Autodesk Inventor part; units mm, degrees
ref_plane "YZ Plane" through (0, 0, 0) normal (1, 0, 0) x (0, 1, 0)
ref_plane "XZ Plane" through (0, 0, 0) normal (0, 1, 0) x (-1, 0, 0)
ref_plane "XY Plane" through (0, 0, 0) normal (0, 0, 1) x (1, 0, 0)
sketch "Block1" plane through (0, 0, 0) normal (0, 0, 1) x (1, 0, 0)
  circle A0 centre (74.029, 24.2723) radius 1
  line L0 (49.279, 30.4723) -> (71.779, 30.4723)
  line L1 (71.779, 30.4723) -> (71.779, 18.0723)
  line L2 (71.779, 18.0723) -> (49.279, 18.0723)
  line L3 (49.279, 18.0723) -> (49.279, 30.4723)
  line L4 (49.279, 30.4723) -> (44.779, 30.4723)
  line L5 (44.779, 30.4723) -> (44.779, 18.0723)
  line L6 (44.779, 18.0723) -> (49.279, 18.0723)
  line L7 (49.279, 18.0723) -> (49.279, 30.4723)
  line L8 (71.779, 30.4723) -> (76.279, 30.4723)
  line L9 (76.279, 30.4723) -> (76.279, 18.0723)
  line L10 (76.279, 18.0723) -> (71.779, 18.0723)
  line L11 (71.779, 18.0723) -> (71.779, 30.4723)
  line L12 (44.779, 24.2723) -> (76.279, 24.2723) construction
  line L13 (47.029, 30.4723) -> (47.029, 18.0723) construction
  circle A1 centre (47.029, 24.2723) radius 1
  line L14 (74.029, 30.4723) -> (74.029, 18.0723) construction
  point P0 (60.979, 24.0984)
  dimension "d7" = 22.5
  dimension "d8" = 12.4
  dimension "d9" = 4.5
  dimension "d10" = 4.5
  dimension "d11" = 2
  dimension "d12" = 2
sketch "Sketch1" plane through (0, 0, 0) normal (0, 0, 1) x (1, 0, 0)
  line L0 (-92.7646, -8.503) -> (-89.7646, -8.503)
  line L1 (-89.7646, -8.503) -> (-89.7646, -11.753)
  line L2 (-89.7646, -11.753) -> (-92.7646, -11.753)
  line L3 (-92.7646, -11.753) -> (-92.7646, -8.503)
  line L4 (-92.7646, -21.6527) -> (-89.7646, -21.6527)
  line L5 (-89.7646, -21.6527) -> (-89.7646, -21.7527)
  line L6 (-89.7646, -21.7527) -> (-92.7646, -21.7527)
  line L7 (-92.7646, -21.7527) -> (-92.7646, -21.6527)
  line L8 (-51.3097, 52.8088) -> (28.6903, 52.8088)
  line L9 (28.6903, 52.8088) -> (28.6903, 26.8088)
  line L10 (28.6903, 26.8088) -> (-51.3097, 26.8088)
  line L11 (-51.3097, 26.8088) -> (-51.3097, 52.8088)
  line L12 (-51.3097, 39.8088) -> (28.6903, 39.8088) construction
  line L13 (-21.3097, 46.8088) -> (-18.0597, 46.8088)
  line L14 (-18.0597, 46.8088) -> (-18.0597, 32.8088)
  line L15 (-18.0597, 32.8088) -> (-21.3097, 32.8088)
  line L16 (-21.3097, 32.8088) -> (-21.3097, 46.8088)
  line L17 (-21.3097, 39.8088) -> (-18.0597, 39.8088) construction
  line L18 (-38.3097, 52.8088) -> (-38.3097, 26.8088) construction
  arc A0 (-38.3097, 52.8088) -> (-38.3097, 26.8088) centre (-38.3097, 39.8088) ccw
  line L19 (-11.3097, 52.8088) -> (-11.3097, 26.8088) construction
  line L20 (15.6903, 52.8088) -> (15.6903, 26.8088) construction
  arc A1 (15.6903, 26.8088) -> (15.6903, 52.8088) centre (15.6903, 39.8088) ccw
  point P0 (0, 0)
  dimension "d0" = 3
  dimension "mat" = 3.25
  dimension "d2" = 3
  dimension "d3" = 0.1
  dimension "d23" = 80
  dimension "d24" = 26
  dimension "d29" = 3.25
  dimension "d30" = 14
  dimension "d31" = 30
  dimension "d38" = 13
  dimension "d39" = 13
extrude "Extrusion6" add sketch "Sketch1" along normal blind 3.25 contours L8 A1 L10 A0
equation "\"d29\" = mat"
equation "\"d42\" = mat"
properties part number "arm-servo"
CAD build for the part. Positions are in the model's coordinates, mm. A direction names the side the tool comes from. Give positions to 0.01 mm unless a question says otherwise; leave off trailing zeros. Order: outer loops, then holes, each group sorted by start corner. A loop starts at its lowest first (then second) coordinate and runs counter-clockwise, first axis right, second up.
(1) Saw through at C-C, the plane x = 22.5. Give the cut face in (y, z).
(2) Flat gauge pins, fed straight in: pin 1 (1 mm diameter, centred on y = 41.5, z = 3, fed in from +X); pin 2 (1.6 mm diameter, centred on y = 43, z = 1, fed in from +X); pin 3 (1 mm diameter, centred on y = 41.5, z = 1.5, fed in from -X) (3 decimals). Where does each tip first touch, or does it go through?
(3) Tool access for faces 4 (the flat face through (-12, 40, 0)), 5 (the flat face through (-21.31, 40, 2)): list every direction of +Z, -Z, +X, -X, +Y, -Y with a clear straight run to the whole face (end or side of a thin tool).
(4) Mould opens along Y. For faces 1 (the flat face through (-18.06, 40, 2)), 2 (the cylindrical face through (28.687, 40.095, 1.602)), 3 (the flat face through (-11, 26.809, 2)) say: released by +Y, released by -Y, zero draft, split by the parting line, or undercut.
(5) Drill centre lines: L1, parallel to X at y = 35.5, z = 2.15; L2, parallel to X at y = 45, z = 1.5; L3, parallel to X at y = 50.5, z = 1.15. Where is each one in solid material? Low to high.
(6) Saw through at A-A, the plane z = 2.4. Give the cut face in (x, y).
(7) Saw through at D-D, the plane y = 39.25. Give the cut face in (x, z), then the cut area to 3 significant figures.
(8) Saw through at B-B, the plane y = 43. Give the cut face in (x, z).
Results found:
1. outline: (28.74, 0) - (50.88, 0) - (50.88, 3.25) - (28.74, 3.25) - close
2. pin 1: stops at x = 28.64
2. pin 2: stops at x = 28.47
2. pin 3: stops at x = -51.255
3. face 4: -Z, +X, -X, +Y, -Y
3. face 5: +Z, -Z
4. face 1: undercut
4. face 2: split by the parting line
4. face 3: released by -Y
5. L1: x = -50.57 to -21.31, -18.06 to 27.96
5. L2: x = -50.23 to -21.31, -18.06 to 27.61
5. L3: x = -45.71 to 23.09
6. outline: (-38.31, 26.81) - (15.69, 26.81) arc R13 ccw to (15.69, 52.81) - (-38.31, 52.81) arc R13 ccw to start; hole (-21.31, 32.81) - (-18.06, 32.81) - (-18.06, 46.81) - (-21.31, 46.81) - close
7. outline: (-51.3, 0) - (-21.31, 0) - (-21.31, 3.25) - (-51.3, 3.25) - close; (-18.06, 0) - (28.68, 0) - (28.68, 3.25) - (-18.06, 3.25) - close
7. area: 249 mm2
8. outline: (-50.91, 0) - (-21.31, 0) - (-21.31, 3.25) - (-50.91, 3.25) - close; (-18.06, 0) - (28.29, 0) - (28.29, 3.25) - (-18.06, 3.25) - close
